```python
from build123d import *

# Parameters (mm, degrees)
SKETCH_1_W          = 112
SKETCH_1_H          = 24
EXTRUDE_1_DEPTH     = 8
SKETCH_2_R          = 1.3
CUT_EXTRUDE_1_DEPTH = 30
SKETCH_3_R          = 2.45
CUT_EXTRUDE_2_DEPTH = 30
CUT_EXTRUDE_3_DEPTH = 2
SKETCH_5_R          = 4.7
CUT_EXTRUDE_4_DEPTH = 1


with BuildPart() as part:
    # 草图1 → 凸台-拉伸1 (new body)
    with BuildSketch(Plane.XY):
        Rectangle(SKETCH_1_W, SKETCH_1_H)
    extrude(amount=EXTRUDE_1_DEPTH)

    # 草图2 → 切除-拉伸1 (cut)
    with BuildSketch(Plane(origin=(0, 12, 0), x_dir=(1, 0, 0), z_dir=(0, 1, 0))):
        with Locations(Location((-15, -4, 0), (0, 0, 270))):
            Circle(SKETCH_2_R)
        with Locations(Location((-45, -4, 0), (0, 0, 270))):
            Circle(SKETCH_2_R)
        with Locations(Location((45, -4, 0), (0, 0, 270))):
            Circle(SKETCH_2_R)
        with Locations(Location((15, -4, 0), (0, 0, 270))):
            Circle(SKETCH_2_R)
    extrude(amount=-CUT_EXTRUDE_1_DEPTH, mode=Mode.SUBTRACT)

    # 草图3 → 切除-拉伸2 (cut)
    with BuildSketch(Plane(origin=(0, 0, 0), x_dir=(-1, 0, 0), z_dir=(0, 0, -1))):
        Circle(SKETCH_3_R)
    extrude(amount=-CUT_EXTRUDE_2_DEPTH, mode=Mode.SUBTRACT)

    # 草图4 → 切除-拉伸3 (cut)
    with BuildSketch(Plane(origin=(0, 0, 0), x_dir=(-1, 0, 0), z_dir=(0, 0, -1))):
        Polygon((4.052179536, -1.964647808), (3.727524679, 2.526966514), (-0.324654856, 4.491614323), (-4.052179536, 1.964647808), (-3.727524679, -2.526966514), (0.324654856, -4.491614323), align=None)
    extrude(amount=-CUT_EXTRUDE_3_DEPTH, mode=Mode.SUBTRACT)

    # 草图5 → 切除-拉伸4 (cut)
    with BuildSketch(Plane.XY.offset(8)):
        Circle(SKETCH_5_R)
    extrude(amount=-CUT_EXTRUDE_4_DEPTH, mode=Mode.SUBTRACT)


solid = part.part
```
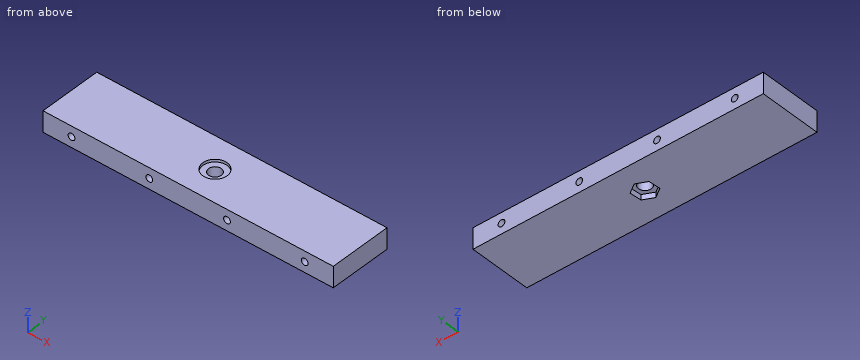
For this review, take the finished solid that the model builds, in its own axes (mm). Give positions to 0.01 mm unless a question says otherwise; leave off trailing zeros. Order: outer loops, then holes, each group sorted by start corner. A loop starts at its lowest first (then second) coordinate and runs counter-clockwise, first axis right, second up.
1) Insertion check: pin 1 (3 mm diameter, centred on x = -45, z = 4, fed in from +Y); pin 2 (4.5 mm diameter, centred on x = 0, y = 0, fed in from +Z); pin 3 (3 mm diameter, centred on x = -1.5, y = 1, fed in from +Z). Each pin has a flat end and moves straight along its axis. Give the tip position at first contact, or say it passes through.
2) Take a section at A-A (z = 4). Give the boundary of the cut face in (x, y), then the cut area to 3 significant figures.
3) Take a section at D-D (y = 9.5). Give the boundary of the cut face in (x, z).
4) Take a section at B-B (x = 15). Give the boundary of the cut face in (y, z), then the cut area to 3 significant figures.
5) Take a section at C-C (y = 0). Give the boundary of the cut face in (x, z).
6) Wall thickness on line 1 (Y direction, x = 0, z = 4.45); line 2 (Y direction, x = 1.5, z = 4.25); line 3 (X direction, y = -2, z = 4): over which ranges is each line inside the solid? List them lowest first.
Derived:
1. pin 1: stops at y = 12
1. pin 2: passes through
1. pin 3: stops at z = 7
2. outline: (-56, -12) - (-46.3, -12) - (-46.3, 12) - (-56, 12) - close; (-43.7, -12) - (-16.3, -12) - (-16.3, 12) - (-43.7, 12) - close; (-13.7, -12) - (13.7, -12) - (13.7, 12) - (-13.7, 12) - close; (16.3, -12) - (43.7, -12) - (43.7, 12) - (16.3, 12) - close; (46.3, -12) - (56, -12) - (56, 12) - (46.3, 12) - close; hole circle Ø4.9 at (0, 0)
2. area: 2,420 mm2
3. outline: (-56, 0) - (56, 0) - (56, 8) - (-56, 8) - close; hole circle Ø2.6 at (-45, 4); hole circle Ø2.6 at (-15, 4); hole circle Ø2.6 at (15, 4); hole circle Ø2.6 at (45, 4)
4. outline: (-12, 0) - (12, 0) - (12, 2.7) - (-12, 2.7) - close; (-12, 5.3) - (12, 5.3) - (12, 8) - (-12, 8) - close
4. area: 130 mm2
5. outline: (-56, 0) - (-3.91, 0) - (-3.91, 2) - (-2.45, 2) - (-2.45, 7) - (-4.7, 7) - (-4.7, 8) - (-56, 8) - close; (2.45, 2) - (3.91, 2) - (3.91, 0) - (56, 0) - (56, 8) - (4.7, 8) - (4.7, 7) - (2.45, 7) - close; hole circle Ø2.6 at (-45, 4); hole circle Ø2.6 at (-15, 4); hole circle Ø2.6 at (15, 4); hole circle Ø2.6 at (45, 4)
6. line 1: y = -12 to -2.45, 2.45 to 12
6. line 2: y = -12 to -1.94, 1.94 to 12
6. line 3: x = -56 to -46.3, -43.7 to -16.3, -13.7 to -1.42, 1.42 to 13.7, 16.3 to 43.7, 46.3 to 56
